Check sheet for the modelled part. Datum: model origin and axes. Units: mm. A direction names the side the tool comes from. Coordinates: 2 decimals unless noted, no trailing zeros. Loops run counter-clockwise (first coordinate to the right, second up) from the corner with the lowest first, then second, coordinate; pieces in that order, holes last. Notation, with made-up numbers: M 88.25,82 L 108.25,82 A15 ccw 108.25,97 Z; hole C 30.25,-29 d8. An arc over 180 degrees is marked long. Answer in a Markdown table with one row per item. Add a question column.
```python
from build123d import *

# Parameters (mm, degrees)
DODANIE_WYCI_GNI_CIE1_DEPTH = 3
DODANIE_WYCI_GNI_CIE2_DEPTH = 51
DODANIE_WYCI_GNI_CIE3_START = -5
DODANIE_WYCI_GNI_CIE3_DEPTH = 5
SZKIC4_R                    = 1.7
WYTNIJ_WYCI_GNI_CIE1_DEPTH  = 5
SZKIC5_R                    = 6.5
SZKIC5_R_2                  = 1.7
WYTNIJ_WYCI_GNI_CIE2_DEPTH  = 5


with BuildPart() as part:
    # Szkic1 → Dodanie-wyciągnięcie1 (new body)
    with BuildSketch(Plane(origin=(0, 0, 0), x_dir=(1, 0, 0), z_dir=(0, 1, 0))):
        with BuildLine():
            Line((-27.5, 20), (-12.5, 20))
            ThreePointArc((-12.5, 20), (-11.934314575, 20.040202025), (-11.38, 20.16))
            ThreePointArc((-11.38, 20.16), (15.5, 0), (-11.38, -20.16))
            ThreePointArc((-11.38, -20.16), (-11.934314575, -20.040202025), (-12.5, -20))
            Line((-12.5, -20), (-27.5, -20))
            Line((-27.5, -20), (-27.5, -31))
            ThreePointArc((-27.5, -31), (-26.328427125, -33.828427125), (-23.5, -35))
            Line((-23.5, -35), (23.5, -35))
            ThreePointArc((23.5, -35), (26.328427125, -33.828427125), (27.5, -31))
            Line((27.5, -31), (27.5, 31))
            ThreePointArc((27.5, 31), (26.328427125, 33.828427125), (23.5, 35))
            Line((23.5, 35), (-23.5, 35))
            ThreePointArc((-23.5, 35), (-26.328427125, 33.828427125), (-27.5, 31))
            Line((-27.5, 31), (-27.5, 20))
        make_face()
    extrude(amount=DODANIE_WYCI_GNI_CIE1_DEPTH)

    # Szkic2 → Dodanie-wyciągnięcie2 (add)
    with BuildSketch(Plane(origin=(0, 3, 0), x_dir=(1, 0, 0), z_dir=(0, 1, 0))):
        with BuildLine():
            Line((-12.5, -20), (-23.638357147, -20))
            ThreePointArc((-23.638357147, -20), (21.5, 0), (-23.638357147, 20))
            Line((-23.638357147, 20), (-12.5, 20))
            ThreePointArc((-12.5, 20), (-11.934314575, 20.040202025), (-11.38, 20.16))
            ThreePointArc((-11.38, 20.16), (15.5, 0), (-11.38, -20.16))
            ThreePointArc((-11.38, -20.16), (-11.934314575, -20.040202025), (-12.5, -20))
        make_face()
    extrude(amount=DODANIE_WYCI_GNI_CIE2_DEPTH)

    # Szkic3 → Dodanie-wyciągnięcie3 (add)
    with BuildSketch(Plane(origin=(0, 54, 0), x_dir=(1, 0, 0), z_dir=(0, 1, 0)).offset(DODANIE_WYCI_GNI_CIE3_START)):
        with BuildLine():
            Line((-23.638357147, 20), (-23.638357147, -20))
            ThreePointArc((-23.638357147, -20), (21.5, 0), (-23.638357147, 20))
        make_face()
    extrude(amount=DODANIE_WYCI_GNI_CIE3_DEPTH)

    # Szkic4 → Wytnij-wyciągnięcie1 (cut)
    with BuildSketch(Plane(origin=(0, 3, 0), x_dir=(1, 0, 0), z_dir=(0, 1, 0))):
        with Locations(Location((-21.5, -30, 0), (0, 0, 270))):
            Circle(SZKIC4_R)
        with Locations(Location((21.5, -30, 0), (0, 0, 270))):
            Circle(SZKIC4_R)
        with Locations(Location((21.5, 30, 0), (0, 0, 270))):
            Circle(SZKIC4_R)
        with Locations(Location((-21.5, 30, 0), (0, 0, 270))):
            Circle(SZKIC4_R)
        with Locations(Location((6.5, -30, 0), (0, 0, 270))):
            Circle(SZKIC4_R)
        with Locations(Location((6.5, 30, 0), (0, 0, 270))):
            Circle(SZKIC4_R)
    extrude(amount=-WYTNIJ_WYCI_GNI_CIE1_DEPTH, mode=Mode.SUBTRACT)

    # Szkic5 → Wytnij-wyciągnięcie2 (cut)
    with BuildSketch(Plane(origin=(0, 54, 0), x_dir=(1, 0, 0), z_dir=(0, 1, 0))):
        with Locations(Location((-12.5, 0, 0), (0, 0, 270))):
            Circle(SZKIC5_R)
        with Locations(Location((-5.5, -15.5, 0), (0, 0, 270))):
            Circle(SZKIC5_R_2)
        with Locations(Location((-18.923393759, -7.75, 0), (0, 0, 270))):
            Circle(SZKIC5_R_2)
        with Locations(Location((-18.923393759, 7.75, 0), (0, 0, 270))):
            Circle(SZKIC5_R_2)
        with Locations(Location((-5.5, 15.5, 0), (0, 0, 270))):
            Circle(SZKIC5_R_2)
        with Locations(Location((7.923393759, 7.75, 0), (0, 0, 270))):
            Circle(SZKIC5_R_2)
        with Locations(Location((7.923393759, -7.75, 0), (0, 0, 270))):
            Circle(SZKIC5_R_2)
    extrude(amount=-WYTNIJ_WYCI_GNI_CIE2_DEPTH, mode=Mode.SUBTRACT)


solid = part.part
```
Q1. Cross-section at D-D (y = 31.5). Record the cut outline in (x, z).
Q2. Go/stop test with flat-tipped pins: pin 1 (2 mm diameter, centred on x = 2, y = 46, fed in from -Z); pin 2 (1.5 mm diameter, centred on y = 21, z = 11.5, fed in from +X); pin 3 (1 mm diameter, centred on y = 35.5, z = 1, fed in from -X). Record where each tip stops, or that it passes through.
Q3. Cross-section at B-B (z = -7.75). Record the cut outline in (x, y), plus the area to 3 significant figures.
Q4. Thickness scan on L1, parallel to X at y = 1.7, z = 30; L2, parallel to Z at x = -5.5, y = 29.5; L3, parallel to Z at x = -15, y = 2.5. Record the ranges inside material, lowest first.
Q5. Cross-section at A-A (z = -30). Record the cut outline in (x, y).
Q6. Cross-section at C-C (x = -15.5). Record the cut outline in (y, z).
Q7. Access from +Z, -Z, +X, -X, +Y, -Y to the whole of each face (thin tool, end or side, straight path). Record for faces 1 (the face through (15.493, 24.157, -0.545)), 2 (the face through (6.264, 51.535, 7.381)).
Q8. Mould release check, pull along X, two halves, no side actions. Record for faces 3 (the face through (-18, 24, 20)), 4 (the face through (-27.5, 1, 25)), 5 (the face through (-20.99, 1.52, -28.38)), 6 (the face through (-17.238, 51.535, 7.529)): released by +X, released by -X, zero draft, split by the parting line, or undercut.
Answer key:
| question | item | result |
|---|---|---|
| 1 | outline | M -23.64,-20 A27 ccw long -23.64,20 L -12.5,20 A4 ccw -11.38,20.16 A21 cw long -11.38,-20.16 A4 ccw -12.5,-20 Z |
| 2 | pin 1 | z = -26.21 |
| 2 | pin 2 | x = 19.27 |
| 2 | pin 3 | x = 15.45 |
| 3 | outline | M -23.64,49 L -20.62,49 L -20.62,54 L -23.64,54 Z; M -17.22,49 L 6.22,49 L 6.22,54 L -17.22,54 Z; M 9.62,49 L 14.02,49 L 14.02,0 L 27.5,0 L 27.5,3 L 20.36,3 L 20.36,54 L 9.62,54 Z |
| 3 | area | 518 mm^2 |
| 4 | L1 | -27.5 to -23.2, -19.8 to 4.8, 8.2 to 19.8, 23.2 to 27.5 |
| 4 | L2 | -27 to -21, 21 to 27 |
| 4 | L3 | -35 to -20, 20 to 35 |
| 5 | outline | M -27.5,0 L -23.2,0 L -23.2,3 L -27.5,3 Z; M -19.8,0 L 4.8,0 L 4.8,3 L -19.8,3 Z; M 8.2,0 L 19.8,0 L 19.8,3 L 8.2,3 Z; M 23.2,0 L 27.5,0 L 27.5,3 L 23.2,3 Z |
| 6 | outline | M 0,-35 L 3,-35 L 3,-25.08 L 54,-25.08 L 54,-5.77 L 49,-5.77 L 49,-20 L 0,-20 Z; M 0,20 L 49,20 L 49,5.77 L 54,5.77 L 54,25.08 L 3,25.08 L 3,35 L 0,35 Z |
| 7 | face 1 | -Y |
| 7 | face 2 | +Y, -Y |
| 8 | face 3 | zero draft |
| 8 | face 4 | released by -X |
| 8 | face 5 | undercut |
| 8 | face 6 | undercut |
